Autodesk Inventor part; units mm, degrees
ref_plane "YZ Plane" through (0, 0, 0) normal (1, 0, 0) x (0, 1, 0)
ref_plane "XZ Plane" through (0, 0, 0) normal (0, 1, 0) x (-1, 0, 0)
ref_plane "XY Plane" through (0, 0, 0) normal (0, 0, 1) x (1, 0, 0)
sketch "Sketch1" plane through (0, 0, 0) normal (0, 1, 0) x (-1, 0, 0)
  line L0 (-44.45, -63.5) -> (44.45, -63.5)
  line L1 (44.45, -63.5) -> (44.45, 63.5)
  line L2 (44.45, 63.5) -> (-44.45, 63.5)
  line L3 (-44.45, 63.5) -> (-44.45, -63.5)
  line L4 (-44.45, -63.5) -> (44.45, 63.5) construction
  line L5 (44.45, -63.5) -> (-44.45, 63.5) construction
  point P0 (0, 0)
  dimension "d0" = 127
  dimension "d1" = 88.9
extrude "Extrusion1" add sketch "Sketch1" along normal blind 12.7
sketch "Sketch2" plane through (0, 12.7, 0) normal (0, 1, 0) x (1, 0, 0)
  line L0 (44.45, 63.5) -> (-44.45, 63.5)
  line L1 (-44.45, 63.5) -> (-44.45, -63.5)
  line L2 (44.45, 63.5) -> (-44.45, 63.5)
  line L3 (-44.45, 63.5) -> (-44.45, -41.275)
  line L4 (-44.45, -41.275) -> (44.45, -41.275)
  line L5 (44.45, -41.275) -> (44.45, 63.5)
  point P0 (0, 0)
  dimension "d4" = 104.775
extrude "Extrusion2" add sketch "Sketch2" along normal blind 38.1
sketch "Sketch4" plane through (-44.45, 0, -63.5) normal (-1, 0, 0) x (0, 0, 1)
  line L0 (101.6, 47.625) -> (3.175, 47.625)
  line L1 (3.175, 47.625) -> (3.175, 12.7)
  line L2 (3.175, 12.7) -> (101.6, 12.7)
  line L3 (101.6, 12.7) -> (101.6, 47.625)
  line L4 (0, 0) -> (0, 50.8)
  line L5 (0, 50.8) -> (104.775, 50.8)
  line L6 (104.775, 12.7) -> (104.775, 50.8)
  line L7 (0, 0) -> (127, 0)
  point P0 (63.5, 0)
  dimension "d11" = 3.175
  dimension "d12" = 3.175
  dimension "d13" = 3.175
  dimension "d14" = 12.7
extrude "Extrusion3" cut sketch "Sketch4" against normal blind 85.725
sketch "Sketch5" plane through (0, 50.8, 0) normal (0, 1, 0) x (1, 0, 0)
  line L0 (-44.45, 63.5) -> (-44.45, -41.275)
  line L1 (44.45, -63.5) -> (44.45, 63.5)
  line L2 (-44.45, -28.575) -> (44.45, -28.575)
  line L3 (44.45, -28.575) -> (44.45, 50.8)
  line L4 (44.45, 50.8) -> (-44.45, 50.8)
  line L5 (-44.45, 50.8) -> (-44.45, -28.575)
  line L6 (44.45, 63.5) -> (-44.45, 63.5)
  line L7 (-44.45, -41.275) -> (44.45, -41.275)
  point P0 (0, 0)
  dimension "d17" = 12.7
  dimension "d18" = 12.7
extrude "Extrusion4" cut sketch "Sketch5" against normal blind 31.75 contours L4 L1 L2 L0
sketch "Sketch6" plane through (0, 12.7, 0) normal (0, 1, 0) x (1, 0, 0)
  line L0 (44.45, -63.5) -> (44.45, -41.275)
  point P0 (0, 0)
  point P1 (-24.4718, -51.1375)
  point P2 (26.3282, -51.1375)
  dimension "d21" = 50.8
hole "Hole1" at (-24.4718, 12.7, 51.1375) at (26.3282, 12.7, 51.1375) direction (0, -1, 0) diameter 6.7564 end through all
properties part number "KVM Holder"
For this review, take the finished solid that the model builds, in its own axes (mm). A direction names the side the tool comes from. Coordinates: 2 decimals unless noted, no trailing zeros. Loops run counter-clockwise (first coordinate to the right, second up) from the corner with the lowest first, then second, coordinate; pieces in that order, holes last.
1. Add section C-C, the plane x = -15. Give the boundary of the cut face in (y, z) (3 decimals).
2. Mouldability with a two-part tool opening along Y and no side actions: class faces 1 (the flat face through (41.275, 18.8, -11.8)), 2 (the flat face through (-2, 47.625, 33)), 3 (the flat face through (1, 12.7, 53)), 4 (the cylindrical face through (25.31, 6.26, 54.36)) as +Y half, -Y half, draft (parallel to the pull), parting line (faces both ways), or undercut.
3. Insertion check: P1, Ø3.5, axis at x = 43, z = -28, coming from the +Y side; P2, Ø11, axis at x = -24.47, z = 51.14, coming from the +Y side; P3, Ø10, axis at x = -3.5, y = 43.5, coming from the +Z side (3 decimals); P4, Ø7.5, axis at x = 19.5, z = -54, coming from the -Y side. Each pin has a flat end and moves straight along its axis. Give the tip position at first contact, or say it passes through.
4. Add section D-D, the plane z = -2. Give the boundary of the cut face in (x, y) (3 decimals), then the cut area to 3 significant figures.
5. For faces 5 (the flat face through (-2, 47.625, -55)), 6 (the flat face through (43, 19.05, -12)), 7 (the flat face through (-1, 31, 41.275)), 8 (the flat face through (-44.45, 10, -5)), 9 (the cylindrical face through (-25.49, 6.26, 54.36)), list the 3-axis set-ups (+Z, -Z, +X, -X, +Y, -Y) from which the entire face can be reached by the end or side of a thin tool; tool diameter is ignored.
6. For line 1 (Z direction, x = -12.5, y = 40) (3 decimals); line 2 (Y direction, x = 2.5, z = 33) (3 decimals); line 3 (Y direction, x = -19, z = -37), list the stretches that pass through material, from the lowest coordinate up.
7. Add section A-A, the plane y = 24.5. Give the boundary of the cut face in (x, z) (3 decimals), then the cut area to 3 significant figures.
8. Add section B-B, the plane z = 35.5. Give the boundary of the cut face in (x, y) (3 decimals), then the cut area to 3 significant figures.
Result:
1. outline: (0, -63.5) - (50.8, -63.5) - (50.8, -50.8) - (47.625, -50.8) - (47.625, -60.325) - (12.7, -60.325) - (12.7, 38.1) - (47.625, 38.1) - (47.625, 28.575) - (50.8, 28.575) - (50.8, 41.275) - (12.7, 41.275) - (12.7, 63.5) - (0, 63.5) - close
2. face 1: undercut
2. face 2: undercut
2. face 3: +Y half
2. face 4: draft
3. P1: stops at y = 19.05
3. P2: stops at y = 12.7
3. P3: stops at z = 41.275
3. P4: stops at y = 0
4. outline: (-44.45, 0) - (44.45, 0) - (44.45, 19.05) - (41.275, 19.05) - (41.275, 12.7) - (-44.45, 12.7) - close
4. area: 1,150 mm2
5. face 5: -X
5. face 6: +X, -X, +Y
5. face 7: +Z, +X, -X, +Y
5. face 8: +Z, -Z, -X, +Y, -Y
5. face 9: +Y, -Y
6. line 1: z = -63.5 to -60.325, 38.1 to 41.275
6. line 2: y = 0 to 12.7, 47.625 to 50.8
6. line 3: y = 0 to 12.7
7. outline: (-44.45, -63.5) - (44.45, -63.5) - (44.45, -50.8) - (41.275, -50.8) - (41.275, -60.325) - (-44.45, -60.325) - close; (-44.45, 38.1) - (41.275, 38.1) - (41.275, 28.575) - (44.45, 28.575) - (44.45, 41.275) - (-44.45, 41.275) - close
7. area: 625 mm2
8. outline: (-44.45, 0) - (44.45, 0) - (44.45, 50.8) - (-44.45, 50.8) - (-44.45, 47.625) - (41.275, 47.625) - (41.275, 12.7) - (-44.45, 12.7) - close
8. area: 1,520 mm2
